Study the drawing (mm; zero at the part's minimum x, y, z) and answer. A direction names the side the tool comes from. Round coordinates to 2 decimals unless told otherwise and drop trailing zeros. Order: outer loops, then holes, each group sorted by start corner. A loop starts at its lowest first (then second) coordinate and runs counter-clockwise, first axis right, second up. Notation, with made-up numbers: (58, 81) -> (80, 81) arc R18 ccw to (80, 92) -> close; hole circle Ø5 at (5.25, 0.25). An arc over 180 degrees is marked (long way). Answer in a Markdown table with one row per item. Add a question column.
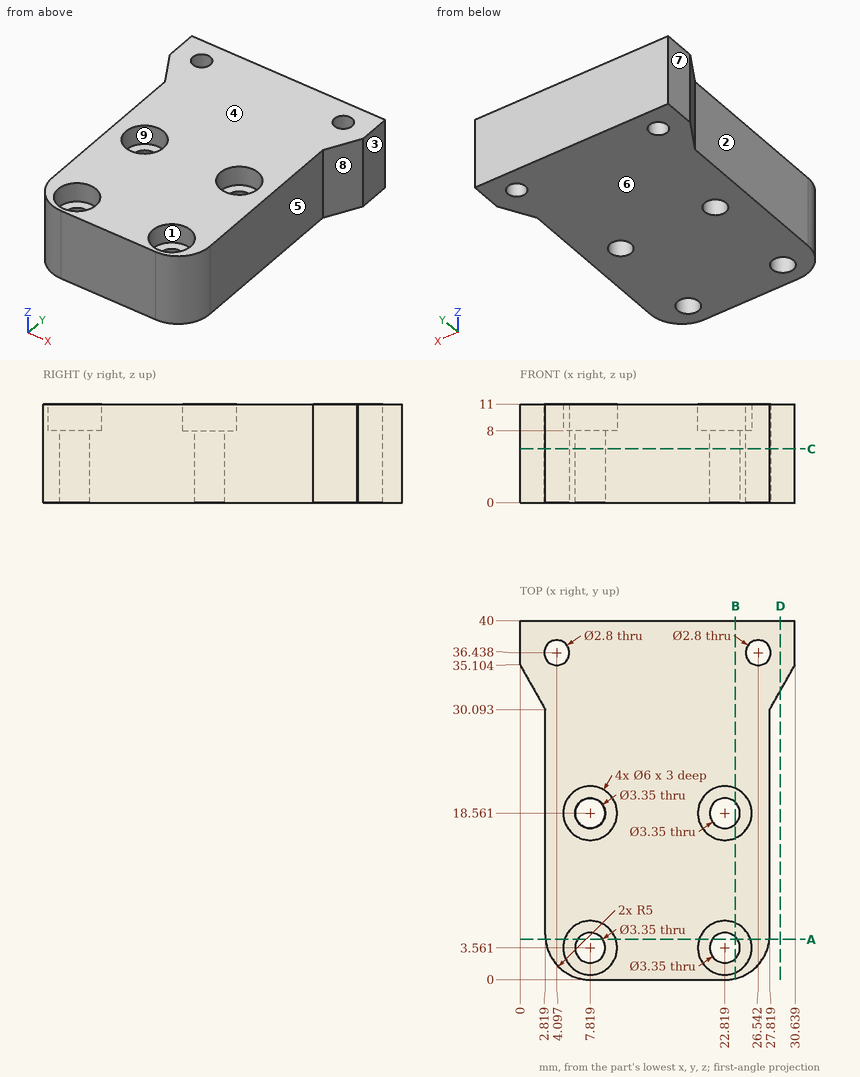
Item 1: The part is cut by section A-A, the plane y = 4.5. Give the vertices of the cut face in (x, z) (1 decimal).
Item 2: The part is cut by section B-B, the plane x = 24. Give the vertices of the cut face in (y, z).
Item 3: The part is cut by section C-C, the plane z = 6. State how many separate pieces and enclosed holes the cut face has.
Item 4: Flat-ended cylindrical pins translate along their axes: P1, Ø5, axis at x = 7.82, y = 3.56, coming from the +Z side; P2, Ø2, axis at x = 26.5, z = 9.5, coming from the -Y side; P3, Ø3, axis at x = 22.82, y = 3.56, coming from the -Z side; P4, Ø5.5, axis at y = 14, z = 4, coming from the +X side. Find the tip coordinate at first contact, or state that the pin passes through.
Item 5: A tool of negligible diameter and unlimited length cuts with its end or side. For the marked faces 1, 2, 3, 4 and 5, from which of +Z, -Z, +X, -X, +Y, -Y can it reach the whole face along a straight path? Write none if from no direction.
Item 6: For a pull along X with two mould halves and no side action, classify the marked faces 6, 7, 8 and 9 as released by +X, released by -X, zero draft, split by the parting line, or undercut.
Item 7: Find the intervals of material crossed by probe 1 along Y at (x, z) = (8, 9) (1 decimal); probe 2 along X at (y, z) = (36, 1); probe 3 along X at (y, z) = (37, 9.75) (1 decimal), in increasing order. Write a range as [from, to].
Item 8: The part is cut by section D-D, the plane x = 29. Give the vertices of the cut face in (y, z).
Resolved:
| question | item | result |
|---|---|---|
| 1 | outline | (2.8, 0) -> (6.4, 0) -> (6.4, 8) -> (5, 8) -> (5, 11) -> (2.8, 11) -> close; (9.2, 0) -> (21.4, 0) -> (21.4, 8) -> (20, 8) -> (20, 11) -> (10.7, 11) -> (10.7, 8) -> (9.2, 8) -> close; (24.2, 0) -> (27.8, 0) -> (27.8, 11) -> (25.7, 11) -> (25.7, 8) -> (24.2, 8) -> close |
| 2 | outline | (0.14, 0) -> (2.37, 0) -> (2.37, 8) -> (0.8, 8) -> (0.8, 11) -> (0.14, 11) -> close; (4.75, 0) -> (17.37, 0) -> (17.37, 8) -> (15.8, 8) -> (15.8, 11) -> (6.32, 11) -> (6.32, 8) -> (4.75, 8) -> close; (19.75, 0) -> (40, 0) -> (40, 11) -> (21.32, 11) -> (21.32, 8) -> (19.75, 8) -> close |
| 3 | separate pieces | 1 |
| 3 | enclosed holes | 6 |
| 4 | P1 | z = 8 |
| 4 | P2 | y = 0.78 |
| 4 | P3 | through |
| 4 | P4 | x = 27.82 |
| 5 | face 1 | +Z |
| 5 | face 2 | +Z, -Z, -X, -Y |
| 5 | face 3 | +Z, -Z, +X, +Y, -Y |
| 5 | face 4 | +Z, +X, -X, +Y, -Y |
| 5 | face 5 | +Z, -Z, +X, -Y |
| 6 | face 6 | zero draft |
| 6 | face 7 | released by -X |
| 6 | face 8 | released by +X |
| 6 | face 9 | undercut |
| 7 | probe 1 | [0, 0.6], [6.6, 15.6], [21.6, 40] |
| 7 | probe 2 | [0, 2.77], [5.43, 25.21], [27.87, 30.64] |
| 7 | probe 3 | [0, 2.8], [5.4, 25.3], [27.8, 30.6] |
| 8 | outline | (32.19, 0) -> (40, 0) -> (40, 11) -> (32.19, 11) -> close |
